from build123d import *

# Parameters (mm, degrees)
BOSS_EXTRUDE1_DEPTH = 2
SKETCH3_R           = 1
SKETCH3_R_2         = 1.5
CUT_EXTRUDE1_DEPTH  = 20.787938245
SKETCH4_R           = 4.5
SKETCH4_R_2         = 3.179560916
BOSS_EXTRUDE2_DEPTH = 3
FILLET1_R           = 0.5


with BuildPart() as part:
    # Sketch1 → Boss-Extrude1 (new body)
    with BuildSketch(Plane(origin=(0, 0, 0), x_dir=(1, 0, 0), z_dir=(0, 1, 0))):
        with BuildLine():
            Line((4.472135955, 4), (16.25, 2.5))
            ThreePointArc((16.25, 2.5), (18.75, 0), (16.25, -2.5))
            Line((16.25, -2.5), (4.472135955, -4))
            ThreePointArc((4.472135955, -4), (0, -6), (-4.472135955, -4))
            Line((-4.472135955, -4), (-16.25, -2.5))
            ThreePointArc((-16.25, -2.5), (-18.75, 0), (-16.25, 2.5))
            Line((-16.25, 2.5), (-4.472135955, 4))
            ThreePointArc((-4.472135955, 4), (0, 6), (4.472135955, 4))
        make_face()
    extrude(amount=BOSS_EXTRUDE1_DEPTH)

    # Sketch3 → Cut-Extrude1 (cut, through all)
    with BuildSketch(Plane(origin=(0, 2, 0), x_dir=(1, 0, 0), z_dir=(0, 1, 0))):
        with Locations(Location((-10.25, 0, 0), (0, 0, 270))):
            Circle(SKETCH3_R)
        with Locations(Location((-7.25, 0, 0), (0, 0, 270))):
            Circle(SKETCH3_R)
        with Locations(Location((0, 0, 0), (0, 0, 270))):
            Circle(SKETCH3_R_2)
        with Locations(Location((13.25, 0, 0), (0, 0, 270))):
            Circle(SKETCH3_R)
        with Locations(Location((16.25, 0, 0), (0, 0, 270))):
            Circle(SKETCH3_R)
        with Locations(Location((10.25, 0, 0), (0, 0, 270))):
            Circle(SKETCH3_R)
        with Locations(Location((-16.25, 0, 0), (0, 0, 270))):
            Circle(SKETCH3_R)
        with Locations(Location((-13.25, 0, 0), (0, 0, 270))):
            Circle(SKETCH3_R)
        with Locations(Location((7.25, 0, 0), (0, 0, 90))):
            Circle(SKETCH3_R)
    extrude(amount=-CUT_EXTRUDE1_DEPTH, mode=Mode.SUBTRACT)

    # Sketch4 → Boss-Extrude2 (add)
    with BuildSketch(Plane.XZ):
        with Locations(Location((0, 0, 0), (0, 0, 90))):
            Circle(SKETCH4_R)
        with Locations(Location((0, 0, 0), (0, 0, 270))):
            Circle(SKETCH4_R_2, mode=Mode.SUBTRACT)
    extrude(amount=BOSS_EXTRUDE2_DEPTH)

    # Fillet1
    fillet1_edges = [part.edges().sort_by_distance(p)[0] for p in [
        (0, -3, -4.5),
    ]]
    fillet(fillet1_edges, radius=FILLET1_R)


solid = part.part
For this review, take the finished solid that the model builds, in its own axes (mm). A direction names the side the tool comes from. Round coordinates to 2 decimals unless told otherwise and drop trailing zeros. Loops run counter-clockwise (first coordinate to the right, second up) from the corner with the lowest first, then second, coordinate; pieces in that order, holes last. Notation, with made-up numbers: (6, 48) - (59, 48) arc R8 ccw to (59, 60) - close; hole circle Ø4 at (78, 70.25). An arc over 180 degrees is marked (long way). One line per item, written item: value. Start each with the question number.
Item 1: Take a section at A-A (x = 10.25). Give the boundary of the cut face in (y, z).
Item 2: For faces 1 (the cylindrical face through (-9.26, 1.01, -0.13)), 2 (the flat face through (4.43, 0, -1.42)), list the 3-axis set-ups (+Z, -Z, +X, -X, +Y, -Y) from which the entire face can be reached by the end or side of a thin tool; tool diameter is ignored.
Item 3: For L1, parallel to Y at x = -11, z = -1.75; L2, parallel to Z at x = 17, y = 1.85; L3, parallel to Z at x = 7, y = 1.15, list the stretches that pass through material, from the lowest coordinate up.
Item 4: Take a section at B-B (y = 1.55). State how many separate pieces and enclosed holes the cut face has, plus the area to 3 significant figures.
Item 5: Clearance check with flat-ended pins moving along their axes: pin 1 Ø1.6 at (x, z) = (13.25, 0) entering from -Y; pin 2 Ø1 at (y, z) = (-1, 1.5) entering from +X; pin 3 Ø2 at (x, y) = (-5.5, 1) entering from +Z; pin 4 Ø3 at (x, z) = (16.25, 0) entering from -Y. State where each tip first meets the part, or that it passes through.
Item 6: The part is to be moulded in two halves that separate along Z. For faces 3 (the cylindrical face through (-6.26, 1.01, -0.13)), 4 (the cylindrical face through (0, 1, -6)), 5 (the flat face through (-10.28, 0.99, 3.26)), say which applies: +Z half, -Z half, draft (parallel to the pull), parting line (faces both ways), or undercut.
Item 7: Take a section at C-C (y = -0.4). Give the boundary of the cut face in (x, z).
Answer below:
1. outline: (0, -3.26) - (2, -3.26) - (2, -1) - (0, -1) - close; (0, 1) - (2, 1) - (2, 3.26) - (0, 3.26) - close
2. face 1: +Y, -Y
2. face 2: -Y
3. L1: y = 0 to 2
3. L2: z = -2.38 to -0.66, 0.66 to 2.38
3. L3: z = -3.68 to -0.97, 0.97 to 3.68
4. separate pieces: 1
4. enclosed holes: 9
4. area: 237 mm2
5. pin 1: passes through
5. pin 2: stops at x = 4.39
5. pin 3: stops at z = 4
5. pin 4: stops at y = 0
6. face 3: undercut
6. face 4: -Z half
6. face 5: +Z half
7. outline: circle Ø9 at (0, 0); hole circle Ø6.36 at (0, 0)
